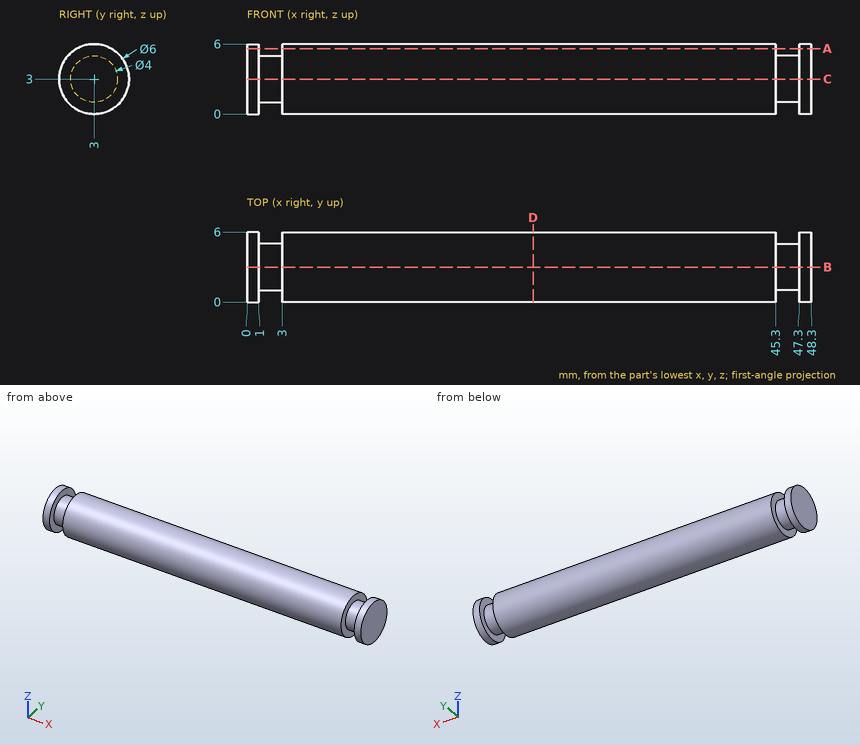
The drawing under review shows one solid part. Ordinate dimensions are in mm from its lowest x, y, z. Coordinates: 2 decimals unless noted, no trailing zeros. Order: outer loops, then holes, each group sorted by start corner. A loop starts at its lowest first (then second) coordinate and runs counter-clockwise, first axis right, second up. Notation, with made-up numbers: (-23.5, 19) -> (-12.5, 19) arc R15 ccw to (-12.5, 33) -> close; hole circle Ø8 at (-38, 56.25). An arc over 180 degrees is marked (long way). Answer in a Markdown table with one row per item. Add a question column.
Item 1: Clearance check with flat-ended pins moving along their axes: pin 1 (1 mm diameter, centred on x = 33, y = 5, fed in from +Z); pin 2 (2 mm diameter, centred on x = 12, y = 4.5, fed in from -Z). State where each tip first meets the part, or that it passes through.
Item 2: We need section D-D on x = 24.5. Write out the cut boundary in (y, z).
Item 3: We need section B-B on y = 3. Write out the cut boundary in (x, z), plus the area to 3 significant figures.
Item 4: We need section A-A on z = 5.6. Write out the cut boundary in (x, y), plus the area to 3 significant figures.
Item 5: To check wall thickness, follow probe 1 along X at (y, z) = (4.8, 4.5); probe 2 along Y at (x, z) = (10, 5.7); probe 3 along Y at (x, z) = (5, 1.45). State the ranges of each line that lie inside material, in increasing order.
Final values:
| question | item | result |
|---|---|---|
| 1 | pin 1 | stops at z = 5.6 |
| 1 | pin 2 | stops at z = 0.04 |
| 2 | outline | circle Ø6 at (3, 3) |
| 3 | outline | (0, 0) -> (1, 0) -> (1, 1) -> (3, 1) -> (3, 0) -> (45.3, 0) -> (45.3, 1) -> (47.3, 1) -> (47.3, 0) -> (48.3, 0) -> (48.3, 6) -> (47.3, 6) -> (47.3, 5) -> (45.3, 5) -> (45.3, 6) -> (3, 6) -> (3, 5) -> (1, 5) -> (1, 6) -> (0, 6) -> close |
| 3 | area | 282 mm2 |
| 4 | outline | (0, 1.5) -> (1, 1.5) -> (1, 4.5) -> (0, 4.5) -> close; (3, 1.5) -> (45.3, 1.5) -> (45.3, 4.5) -> (3, 4.5) -> close; (47.3, 1.5) -> (48.3, 1.5) -> (48.3, 4.5) -> (47.3, 4.5) -> close |
| 4 | area | 133 mm2 |
| 5 | probe 1 | x = 0 to 1, 3 to 45.3, 47.3 to 48.3 |
| 5 | probe 2 | y = 1.69 to 4.31 |
| 5 | probe 3 | y = 0.43 to 5.57 |
